Geometry: final body of the model. Coordinates: model frame, mm. Face numbers are marked on the shaded views. Coordinates: 2 decimals unless noted, no trailing zeros. Loops run counter-clockwise (first coordinate to the right, second up) from the corner with the lowest first, then second, coordinate; pieces in that order, holes last. Notation, with made-up numbers: M -2.75,23.25 L 22.25,23.25 A17 cw 22.25,32.25 Z; hole C 71,-8 d6. An arc over 180 degrees is marked long. Write item = value, one per line. Start each with the question number.
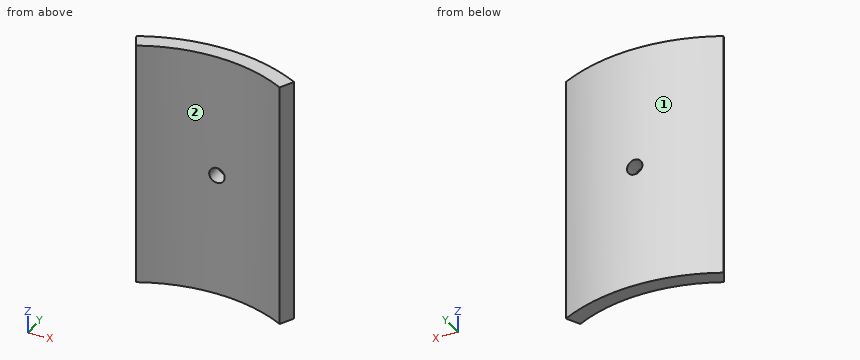
```python
from build123d import *

# Parameters (mm, degrees)
F1_DEPTH = 25.4
F2_R     = 0.79375
F3_DEPTH = 18.8599085


with BuildPart() as f1:
    # F0 (on Top) → F1 (new body)
    with BuildSketch(Plane.XY):
        with BuildLine():
            ThreePointArc((-7.3684509074, 14.5085218531), (0, 16.2724084), (7.3684509074, 14.5085218531))
            Line((7.3684509074, 14.5085218531), (8.0873006024, 15.9239410016))
            ThreePointArc((8.0873006024, 15.9239410016), (0, 17.8599084), (-8.0873006024, 15.9239410016))
            Line((-8.0873006024, 15.9239410016), (-7.3684509074, 14.5085218531))
        make_face()
    extrude(amount=F1_DEPTH)

    # F2 (on Front) → F3 (cut, up to face)
    with BuildSketch(Plane.XZ):
        with Locations((0, 12.7)):
            Circle(F2_R)
    extrude(amount=-F3_DEPTH, mode=Mode.SUBTRACT)


solid = f1.part
```
Item 1: Section query A-A (x = 0). Return the cut outline in (y, z), plus the area to 3 significant figures.
Item 2: Section query D-D (x = -4.75). Return the cut outline in (y, z), plus the area to 3 significant figures.
Item 3: Line query: line 1 (Z direction, x = 0, y = 16.7); line 2 (X direction, y = 14.85, z = 7.75); line 3 (Y direction, x = 0, z = 23.5). Output: solid intervals per line, ascending. Write a range as from..to.
Item 4: Pull-direction query (X, two-part tool) for the marked faces 1 and 2; classes: released by +X, released by -X, zero draft, split by the parting line, or undercut.
Item 5: First-contact query: pin 1 (5 mm diameter, centred on x = -5.5, z = 12.5, fed in from +Y); pin 2 (2 mm diameter, centred on x = 0, z = 12.7, fed in from -Y); pin 3 (6 mm diameter, centred on x = -6, z = 19, fed in from -Y). Flat tips, straight axial feed; report the tip coordinate or a pass-through.
Item 6: Section query C-C (z = 23.5). Return the cut outline in (x, y).
Verdict:
q1.outline = M 16.27,0 L 17.86,0 L 17.86,11.91 L 16.27,11.91 Z; M 16.27,13.49 L 17.86,13.49 L 17.86,25.4 L 16.27,25.4 Z
q1.area = 37.8 mm2
q2.outline = M 15.56,0 L 17.22,0 L 17.22,25.4 L 15.56,25.4 Z
q2.area = 42.0 mm2
q3.line_1 = 0..11.91, 13.49..25.4
q3.line_2 = -7.54..-6.65, 6.65..7.54
q3.line_3 = 16.27..17.86
q4.face_1 = split by the parting line
q4.face_2 = undercut
q5.pin_1 = 17.61
q5.pin_2 = 16.24
q5.pin_3 = 14.51
q6.outline = M -8.09,15.92 L -7.37,14.51 A16.27 cw 7.37,14.51 L 8.09,15.92 A17.86 ccw Z
